from build123d import *

# Parameters (mm, degrees)
BOSS_EXTRUDE1_DEPTH = 30
FILLET1_R           = 1
SHELL1_T            = -2
CUT_EXTRUDE1_REACH  = 48.182
SKETCH3_W           = 10
SKETCH3_H           = 30
BOSS_EXTRUDE2_DEPTH = 30
BOSS_EXTRUDE4_START = -30
BOSS_EXTRUDE4_DEPTH = 30
FILLET2_R           = 3
FILLET3_R           = 1


# Read off the part's stored shape, not the designer's step: Boss-Extrude4
with BuildPart() as part:
    # Sketch1 → Boss-Extrude1 (new body)
    with BuildSketch(Plane(origin=(0, 0, 0), x_dir=(1, 0, 0), z_dir=(0, 1, 0))):
        with BuildLine():
            add(Edge.make_bspline(
                [(-11.25, 10), (-5.781911856, 10.311342007), (10.269870792, 3.454667183), (11.25, 0)],
                knots=[0.452930386, 0.452930386, 0.452930386, 0.452930386, 1, 1, 1, 1], degree=3))
            add(Edge.make_bspline(
                [(-11.25, -10), (-5.781911856, -10.311342007), (10.269870792, -3.454667183), (11.25, 0)],
                knots=[0.452930386, 0.452930386, 0.452930386, 0.452930386, 1, 1, 1, 1], degree=3))
            add(Edge.make_bspline(
                [(-11.25, -10), (-16.718088144, -10.311342007), (-32.769870792, -3.454667183), (-33.75, 0)],
                knots=[0.452930386, 0.452930386, 0.452930386, 0.452930386, 1, 1, 1, 1], degree=3))
            add(Edge.make_bspline(
                [(-11.25, 10), (-16.718088144, 10.311342007), (-32.769870792, 3.454667183), (-33.75, 0)],
                knots=[0.452930386, 0.452930386, 0.452930386, 0.452930386, 1, 1, 1, 1], degree=3))
        make_face()
    extrude(amount=BOSS_EXTRUDE1_DEPTH)

    # Fillet1
    fillet1_edges = [part.edges().sort_by_distance(p)[0] for p in [
        (-33.75, 15, 0),
        (-11.25, 15, -10),
        (11.25, 15, 0),
        (-11.25, 15, 10),
    ]]
    fillet(fillet1_edges, radius=FILLET1_R)

    # Shell1
    shell1_openings = [part.faces().sort_by_distance(p)[0] for p in [
        (-11.25, 30, 0),
        (-11.25, 0, 0),
    ]]
    offset(amount=SHELL1_T, openings=shell1_openings)

    # Sketch3 → Cut-Extrude1 (cut, up to next)
    with BuildSketch(Plane(origin=(0, 0, 0), x_dir=(0, 0, -1), z_dir=(1, 0, 0)), mode=Mode.PRIVATE) as cut_extrude1_sk1:
        with Locations((0, 15)):
            Rectangle(SKETCH3_W, SKETCH3_H)
    cut_extrude1_tool1 = extrude(cut_extrude1_sk1.sketch, amount=CUT_EXTRUDE1_REACH, mode=Mode.PRIVATE) & part.part
    add(cut_extrude1_tool1.solids().sort_by_distance((0, 15, 0))[0], mode=Mode.SUBTRACT)

    # Sketch4 → Boss-Extrude2 (add)
    with BuildSketch(Plane(origin=(0, 30, 0), x_dir=(1, 0, 0), z_dir=(0, 1, 0))):
        with BuildLine():
            Line((4.683590917, 5), (0, 5))
            ThreePointArc((0, 5), (2.341795458, 2.658204542), (4.683590917, 5))
        make_face()
        with BuildLine():
            Line((0, -5), (4.683590917, -5))
            ThreePointArc((4.683590917, -5), (2.341795458, -2.658204542), (0, -5))
        make_face()
    extrude(amount=-BOSS_EXTRUDE2_DEPTH)

    # Boss-Extrude4 outline → Boss-Extrude4 (add)
    with BuildSketch(Plane(origin=(0, 30, 0), x_dir=(1, 0, 0), z_dir=(0, 1, 0)).offset(BOSS_EXTRUDE4_START)):
        with BuildLine():
            ThreePointArc((-27.69069648, -2.46787393), (-28, 0), (-27.69069648, 2.46787393))
            add(Edge.make_bspline(
                [(-27.69069648, 2.46787393), (-27.822031215, 2.39499699), (-27.951900256, 2.322199534), (-28.080260991, 2.249502833), (-28.20707038, 2.176928557), (-28.332284982, 2.10449893), (-28.455860917, 2.032236786), (-28.57775383, 1.960165641), (-28.697918846, 1.88830977), (-28.816310527, 1.816694288), (-28.932882823, 1.745345254), (-29.047589016, 1.674289767), (-29.395924825, 1.455844025), (-29.623125506, 1.309538219), (-29.841540019, 1.164885503), (-30.050742717, 1.022190072), (-30.250257196, 0.881746107), (-30.439599681, 0.743903891), (-30.618272334, 0.609068339), (-30.785746265, 0.477701019), (-30.941461201, 0.350349869), (-31.084828141, 0.227682248), (-31.21523231, 0.110536702), (-31.332067668, -2.7e-08)],
                knots=[0.816861964, 0.816861964, 0.816861964, 0.816861964, 0.816861964, 0.816861964, 0.816861964, 0.816861964, 0.816861964, 0.816861964, 0.816861964, 0.816861964, 0.816861964, 0.853756111, 0.853756111, 0.853756111, 0.853756111, 0.853756111, 0.853756111, 0.853756111, 0.853756111, 0.853756111, 0.853756111, 0.853756111, 0.930801589, 0.930801589, 0.930801589, 0.930801589, 0.930801589, 0.930801589, 0.930801589, 0.930801589, 0.930801589, 0.930801589, 0.930801589, 0.930801589, 0.930801589], degree=12))
            add(Edge.make_bspline(
                [(-27.69069648, -2.46787393), (-27.822031215, -2.39499699), (-27.951900256, -2.322199534), (-28.080260991, -2.249502833), (-28.20707038, -2.176928557), (-28.332284982, -2.10449893), (-28.455860917, -2.032236786), (-28.57775383, -1.960165641), (-28.697918846, -1.88830977), (-28.816310527, -1.816694288), (-28.932882823, -1.745345254), (-29.047589016, -1.674289767), (-29.395924825, -1.455844025), (-29.623125506, -1.309538219), (-29.841540019, -1.164885503), (-30.050742717, -1.022190072), (-30.250257196, -0.881746107), (-30.439599681, -0.743903891), (-30.618272334, -0.609068339), (-30.785746265, -0.477701019), (-30.941461201, -0.350349869), (-31.084828141, -0.227682248), (-31.21523231, -0.110536702), (-31.332067668, -2.7e-08)],
                knots=[0.816861964, 0.816861964, 0.816861964, 0.816861964, 0.816861964, 0.816861964, 0.816861964, 0.816861964, 0.816861964, 0.816861964, 0.816861964, 0.816861964, 0.816861964, 0.853756111, 0.853756111, 0.853756111, 0.853756111, 0.853756111, 0.853756111, 0.853756111, 0.853756111, 0.853756111, 0.853756111, 0.853756111, 0.930801589, 0.930801589, 0.930801589, 0.930801589, 0.930801589, 0.930801589, 0.930801589, 0.930801589, 0.930801589, 0.930801589, 0.930801589, 0.930801589, 0.930801589], degree=12))
        make_face()
    extrude(amount=BOSS_EXTRUDE4_DEPTH)

    # Fillet2
    fillet2_edges = [part.edges().sort_by_distance(p)[0] for p in [
        (-27.69069648, 15, 2.46787393),
        (-27.69069648, 15, -2.46787393),
    ]]
    fillet(fillet2_edges, radius=FILLET2_R)

    # Fillet3
    fillet3_edges = [part.edges().sort_by_distance(p)[0] for p in [
        (4.683590936, 15, -5),
        (4.683590936, 15, 5),
    ]]
    fillet(fillet3_edges, radius=FILLET3_R)


solid = part.part
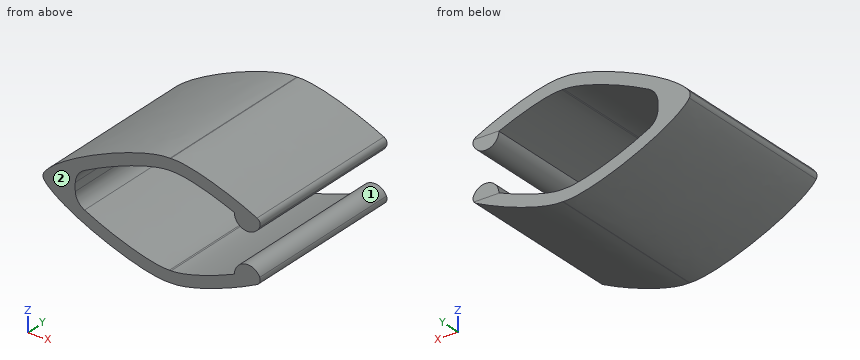
The listing builds one solid part. Answer for the finished solid, in the listing's coordinates (mm). Face numbers are marked on the shaded views. Give positions to 0.01 mm unless a question says otherwise; leave off trailing zeros. One line per question, with ' | ' between items. Start each with the question number.
1. Given pin 1 Ø1 at (x, y) = (-8, 22) entering from +Z, flat-ended and moving along its own axis, determine where the tip first touches the part or whether it passes through.
2. Find the intervals of material crossed by probe 1 along Z at (x, y) = (-17, 6); probe 2 along Z at (x, y) = (-11.5, 19); probe 3 along X at (y, z) = (26, 3.5), in increasing order.
3. For a pull along Z with two mould halves and no side action, classify the marked faces 1 and 2 as pulls with the +Z half, pulls with the -Z half, needs draft (parallel to the pull), parting line crosses it, or undercut.
Response values:
1) pin 1: z = 9.76
2) probe 1: -9.04 to -6.95, 6.95 to 9.04 | probe 2: -10.01 to -8.01, 8.01 to 10.01 | probe 3: -29.9 to -25.71, 0.54 to 4.14
3) face 1: undercut | face 2: needs draft
